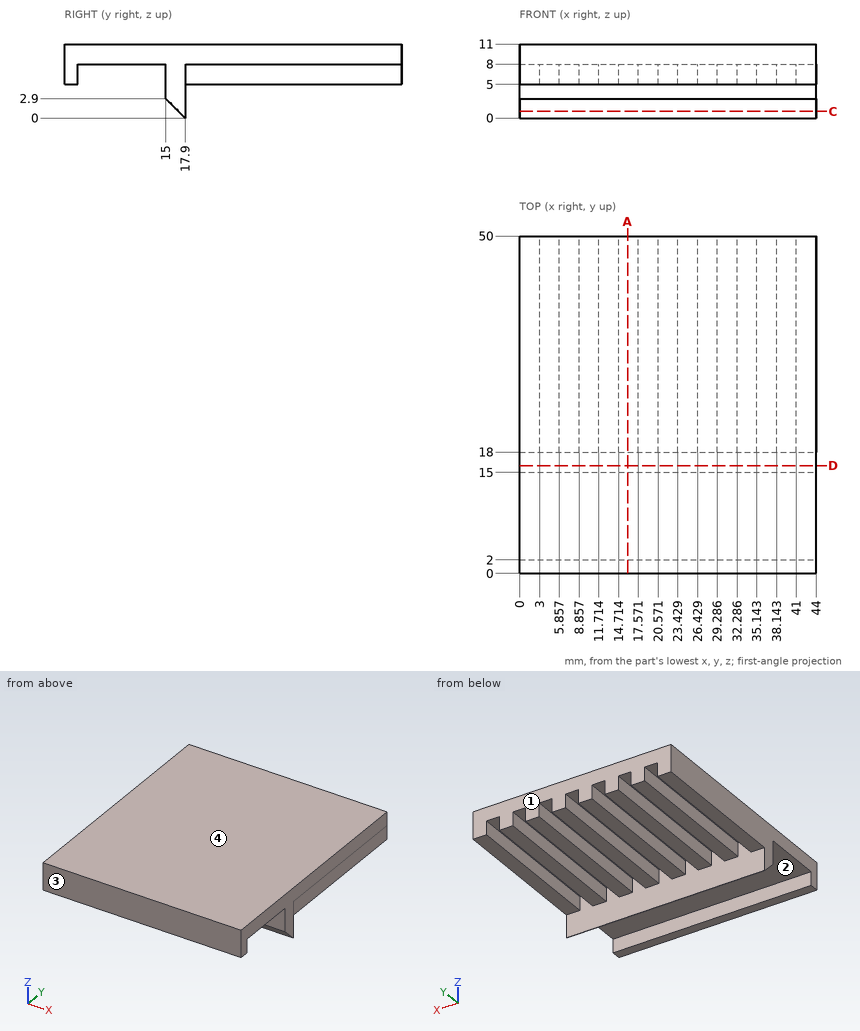
Study the drawing (mm; zero at the part's minimum x, y, z) and answer. Round coordinates to 2 decimals unless told otherwise and drop trailing zeros. Loops run counter-clockwise (first coordinate to the right, second up) from the corner with the lowest first, then second, coordinate; pieces in that order, holes last. Notation, with made-up numbers: (43.5, 41) - (88.5, 41) arc R21 ccw to (88.5, 56) - close; hole circle Ø9 at (51, -22.5). An arc over 180 degrees is marked (long way). Use one line per item in the form item = value. Start each with the question number.
1. Given pin 1 Ø0.9 at (x, y) = (1, 38.5) entering from -Z; pin 2 Ø0.9 at (x, y) = (10.5, 28) entering from -Z; pin 3 Ø1.5 at (y, z) = (31.5, 2.5) entering from -X, each flat-ended and moving along its own axis, determine where each tip first touches the part or whether it passes through.
2. Consider line 1 (Y direction, x = 18.5, z = 5.5); line 2 (Z direction, x = 4.5, y = 10); line 3 (Z direction, x = 14.5, y = 36). Determine where each line is inside the solid, lowest interval first. Write a range as [from, to].
3. For a pull along Y with two mould halves and no side action, classify the marked faces 1, 2, 3 and 4 as pulls with the +Y half, pulls with the -Y half, needs draft (parallel to the pull), parting line crosses it, or undercut.
4. The part is cut by section A-A on x = 16. Determine the outline of the cut face in (y, z), then the cut area to 3 significant figures.
5. The part is cut by section D-D on y = 16. Determine the outline of the cut face in (x, z).
6. The part is cut by section C-C on z = 1. Determine the outline of the cut face in (x, y).
Geometry check:
q1.pin_1 = 5
q1.pin_2 = 8
q1.pin_3 = through
q2.line_1 = [0, 2], [15, 50]
q2.line_2 = [8, 11]
q2.line_3 = [5, 11]
q3.face_1 = pulls with the +Y half
q3.face_2 = undercut
q3.face_3 = pulls with the -Y half
q3.face_4 = needs draft
q4.outline = (0, 5) - (2, 5) - (2, 8) - (15, 8) - (15, 2.9) - (17.9, 0) - (18, 0) - (18, 8) - (50, 8) - (50, 11) - (0, 11) - close
q4.area = 176 mm^2
q5.outline = (0, 1.9) - (44, 1.9) - (44, 11) - (0, 11) - close
q6.outline = (0, 16.9) - (44, 16.9) - (44, 18) - (0, 18) - close
